```python
from build123d import *

# Parameters (mm, degrees)
BOSS_EXTRUDE1_DEPTH = 2.54
SKETCH3_R           = 5.824660453
BOSS_EXTRUDE2_DEPTH = 63.5
BOSS_EXTRUDE3_DEPTH = 123.444
SKETCH5_R           = 1.27
CUT_EXTRUDE1_DEPTH  = 189.695241466
BOSS_EXTRUDE5_DEPTH = 2.54


with BuildPart() as part:
    # Sketch2 → Boss-Extrude1 (new body)
    with BuildSketch(Plane.XY):
        with BuildLine():
            Line((30.943753448, 10.972254104), (83.159468074, -35.423237554))
            ThreePointArc((83.159468074, -35.423237554), (89.122580616, -49.217847067), (82.38831151, -62.652860369))
            Line((82.38831151, -62.652860369), (27.63050793, -106.018808383))
            ThreePointArc((27.63050793, -106.018808383), (22.955852809, -107.34845989), (18.710166876, -104.98318515))
            Line((18.710166876, -104.98318515), (13.979336184, -99.009606578))
            ThreePointArc((13.979336184, -99.009606578), (12.649684678, -94.334951456), (15.014959417, -90.089265524))
            Line((15.014959417, -90.089265524), (53.161684307, -59.878614615))
            ThreePointArc((53.161684307, -59.878614615), (58.933914969, -48.362888928), (53.822675647, -36.538937916))
            Line((53.822675647, -36.538937916), (17.446883148, -4.217771969))
            ThreePointArc((17.446883148, -4.217771969), (15.325686693, 0.154973076), (16.917771969, 4.746883148))
            Line((16.917771969, 4.746883148), (21.979098332, 10.443142925))
            ThreePointArc((21.979098332, 10.443142925), (26.351843377, 12.56433938), (30.943753448, 10.972254104))
        make_face()
    boss_extrude1 = extrude(amount=BOSS_EXTRUDE1_DEPTH)

    # Sketch3 → Boss-Extrude2 (add)
    with BuildSketch(Plane.XY.offset(2.54)):
        with Locations((26.300715817, -94.111678043)):
            Circle(SKETCH3_R)
    boss_extrude2 = extrude(amount=-BOSS_EXTRUDE2_DEPTH)

    # Mirror1: Boss-Extrude1, Boss-Extrude2 across plane
    add(boss_extrude1.mirror(Plane(origin=(26.300715817, -94.111678043, -60.96), x_dir=(1, 0, 0), z_dir=(0, 0, 1))))
    add(boss_extrude2.mirror(Plane(origin=(26.300715817, -94.111678043, -60.96), x_dir=(1, 0, 0), z_dir=(0, 0, 1))))

    # Sketch4 → Boss-Extrude3 (add)
    with BuildSketch(Plane(origin=(0, 0, 0), x_dir=(-1, 0, 0), z_dir=(0, 0, -1))):
        Polygon((-35.247552365, -87.026148251), (-34.459080583, -86.030551823), (-55.688722292, -69.2175411), (-56.477194074, -70.213137529), align=None)
    extrude(amount=BOSS_EXTRUDE3_DEPTH)

    # Sketch5 → Cut-Extrude1 (cut, through all)
    with BuildSketch(Plane(origin=(0, 0, 2.54), x_dir=(-1, 0, 0), z_dir=(0, 0, -1))):
        with Locations(Location((-27.043448187, 0.846577886, 0), (0, 0, 180))):
            Circle(SKETCH5_R)
        with Locations(Location((-34.638461223, -5.901857264, 0), (0, 0, 180))):
            Circle(SKETCH5_R)
    extrude(amount=CUT_EXTRUDE1_DEPTH, mode=Mode.SUBTRACT)

    # Sketch7 → Boss-Extrude5 (add)
    with BuildSketch(Plane.XY.offset(2.54)):
        with BuildLine():
            Line((27.63050793, -106.018808383), (20.056626411, -109.386083488))
            ThreePointArc((20.056626411, -109.386083488), (18.795524409, -109.795283294), (17.476939915, -109.933694534))
            Line((17.476939915, -109.933694534), (6.35, -109.933694534))
            ThreePointArc((6.35, -109.933694534), (1.859871939, -108.073822594), (0, -103.583694534))
            Line((0, -103.583694534), (0, -73.78416115))
            ThreePointArc((0, -73.78416115), (5.031415506, -67.57257239), (12.152388955, -71.204474655))
            Line((12.152388955, -71.204474655), (27.63050793, -106.018808383))
        make_face()
    extrude(amount=-BOSS_EXTRUDE5_DEPTH)


solid = part.part
```
Geometry check sheet. Reference: the model listing, model coordinates, mm. A direction names the side the tool comes from. Give positions to 0.01 mm unless a question says otherwise; leave off trailing zeros. Loops run counter-clockwise (first coordinate to the right, second up) from the corner with the lowest first, then second, coordinate; pieces in that order, holes last. Notation, with made-up numbers: M -19,81.25 L 22,81.25 A16 cw 22,102.25 Z; hole C -2,28 d8. An arc over 180 degrees is marked long. Write item = value, one per line. Start each with the question number.
1. Section check B-B, the plane z = -45. Enter the section's corners in (x, y), plus the area to 3 significant figures.
2. Go/stop test with flat-tipped pins: P1, Ø8, axis at x = 21, z = -106, coming from the -Y side; P2, Ø2, axis at x = 34.64, y = -5.9, coming from the -Z side; P3, Ø10, axis at x = 27, z = -23.5, coming from the -Y side; P4, Ø6, axis at x = 29, z = -74, coming from the +Y side. Record where each tip stops, or that it passes through.
3. Section check A-A, the plane x = 65. Enter the section's corners in (y, z), plus the area to 3 significant figures.
4. Tool access check on faces 5 (the face through (89.127, -49.001, 1.252)), 6 (the face through (46.011, -78.502, -60.107)), 7 (the face through (15.581, -78.917, 1.288)). Record the directions out of +Z, -Z, +X, -X, +Y, -Y that give a thin tool (end or side, any length) a straight path to the whole face; none if there is none.
5. Thickness scan on probe 1 along Z at (x, y) = (44.5, -15); probe 2 along Z at (x, y) = (4.5, -85); probe 3 along X at (y, z) = (-94.5, -103). Record the ranges inside material, lowest first.
6. Section check D-D, the plane x = 48. Enter the section's corners in (y, z), plus the area to 3 significant figures.
7. Draft check along Y on faces 1 (the face through (58.928, -48.549, -123.172)), 2 (the face through (25.542, -88.337, -60.107)), 3 (the face through (35.889, -20.605, 1.252)), 4 (the face through (59, -60, -124.46)). Enter one of: +Y half, -Y half, draft (parallel to the pull), parting line (faces both ways), or undercut.
8. Section check C-C, the plane y = -40.5. Enter the section's corners in (x, z).
Values follow:
q1.outline = C 26.3,-94.11 d11.65; M 34.46,-86.03 L 35.25,-87.03 L 56.48,-70.21 L 55.69,-69.22 Z
q1.area = 141 mm^2
q2.P1 = -99.79
q2.P2 = through
q2.P3 = -99.94
q2.P4 = -88.29
q3.outline = M -76.42,-124.46 L -19.29,-124.46 L -19.29,-121.92 L -76.42,-121.92 Z; M -76.42,0 L -19.29,0 L -19.29,2.54 L -76.42,2.54 Z
q3.area = 290 mm^2
q4.face_5 = +Z, -Z, +X
q4.face_6 = +X, -Y
q4.face_7 = +Z, -Z
q5.probe_1 = -124.46 to -121.92, 0 to 2.54
q5.probe_2 = 0 to 2.54
q5.probe_3 = 20.49 to 32.11
q6.outline = M -89.89,-124.46 L -63.97,-124.46 L -63.97,-121.92 L -75.31,-121.92 L -75.31,0 L -63.97,0 L -63.97,2.54 L -89.89,2.54 L -89.89,0 L -76.93,0 L -76.93,-121.92 L -89.89,-121.92 Z; M -31.37,-124.46 L -4.18,-124.46 L -4.18,-121.92 L -31.37,-121.92 Z; M -31.37,0 L -4.18,0 L -4.18,2.54 L -31.37,2.54 Z
q6.area = 467 mm^2
q7.face_1 = undercut
q7.face_2 = parting line
q7.face_3 = undercut
q7.face_4 = draft
q8.outline = M 57.01,-124.46 L 87.12,-124.46 L 87.12,-121.92 L 57.01,-121.92 Z; M 57.01,0 L 87.12,0 L 87.12,2.54 L 57.01,2.54 Z
